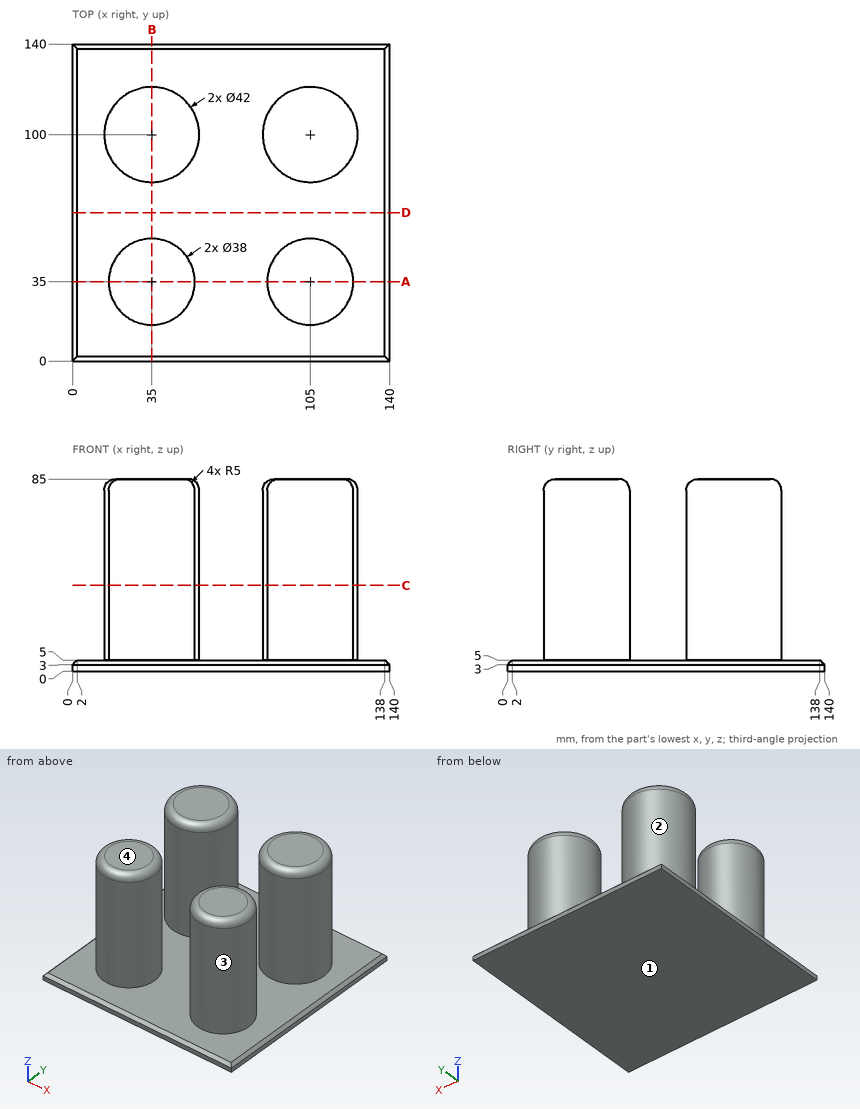
Can you work these out from the drawing? Everything is in mm from the part's minimum corner. A direction names the side the tool comes from. Round coordinates to 2 decimals unless told otherwise and drop trailing zeros. Order: outer loops, then holes, each group sorted by start corner. A loop starts at its lowest first (then second) coordinate and runs counter-clockwise, first axis right, second up. Notation, with made-up numbers: (20.5, 9) - (41.5, 9) arc R33 ccw to (41.5, 45) - close; hole circle Ø2 at (56, -24.5). An arc over 180 degrees is marked (long way). Answer in a Markdown table with one row per item.
(1) Which directions (+Z, -Z, +X, -X, +Y, -Y) give clear straight access to the entire face, cutting with the end or side of a thin tool? Please do the marked faces 1 and 2.
From the geometry:
| item | result |
|---|---|
| face 1 | -Z, +X, -X, +Y, -Y |
| face 2 | +Z |
(2) Suppose I cut it at C-C, the plane z = 38. Please give me the cut outline in (x, y), plus the area to 3 significant figures.
From the geometry:
| item | result |
|---|---|
| outline | circle Ø42 at (35, 100); circle Ø38 at (35, 35); circle Ø42 at (105, 100); circle Ø38 at (105, 35) |
| area | 5,040 mm2 |
(3) For P1, Ø10, axis at y = 97, z = 69.5, coming from the +X side; P2, Ø5, axis at y = 94.5, z = 39.5, coming from the +X side; P3, Ø5, axis at x = 84.5, z = 39, coming from the +Y side; P4, Ø12, axis at x = 98, y = 100, coming from the -Z side, each with a flat end and sliding along its axis, tell me the tip position at first contact or that it passes through.
From the geometry:
| item | result |
|---|---|
| P1 | stops at x = 126 |
| P2 | stops at x = 125.78 |
| P3 | stops at y = 110.82 |
| P4 | stops at z = 0 |
(4) Suppose I cut it at A-A, the plane y = 35. Please give me the cut outline in (x, z).
From the geometry:
| item | result |
|---|---|
| outline | (0, 0) - (140, 0) - (140, 3) - (138, 5) - (124, 5) - (124, 80) arc R5 ccw to (119, 85) - (91, 85) arc R5 ccw to (86, 80) - (86, 5) - (54, 5) - (54, 80) arc R5 ccw to (49, 85) - (21, 85) arc R5 ccw to (16, 80) - (16, 5) - (2, 5) - (0, 3) - close |
(5) Suppose I cut it at B-B, the plane x = 35. Please give me the cut outline in (y, z), plus the area to 3 significant figures.
From the geometry:
| item | result |
|---|---|
| outline | (0, 0) - (140, 0) - (140, 3) - (138, 5) - (121, 5) - (121, 80) arc R5 ccw to (116, 85) - (84, 85) arc R5 ccw to (79, 80) - (79, 5) - (54, 5) - (54, 80) arc R5 ccw to (49, 85) - (21, 85) arc R5 ccw to (16, 80) - (16, 5) - (2, 5) - (0, 3) - close |
| area | 7,070 mm2 |
(6) Suppose I cut it at D-D, the plane y = 65.5. Please give me the cut outline in (x, z).
From the geometry:
| item | result |
|---|---|
| outline | (0, 0) - (140, 0) - (140, 3) - (138, 5) - (2, 5) - (0, 3) - close |
(7) Please list where these lines run through material, in increasing order: L1, parallel to Y at x = 35.5, z = 78; L2, parallel to Z at x = 28, y = 78.5; L3, parallel to Y at x = 90, z = 71. Write a range as from..to.
From the geometry:
| item | result |
|---|---|
| L1 | y = 16.01..53.99, 79.01..120.99 |
| L2 | z = 0..5 |
| L3 | y = 23.34..46.66, 85.3..114.7 |
(8) If we mould it in two halves opening along X, with no side actions, what happens to the marked faces 3 and 4? For each: released by +X, released by -X, zero draft, split by the parting line, or undercut.
From the geometry:
| item | result |
|---|---|
| face 3 | undercut |
| face 4 | zero draft |
